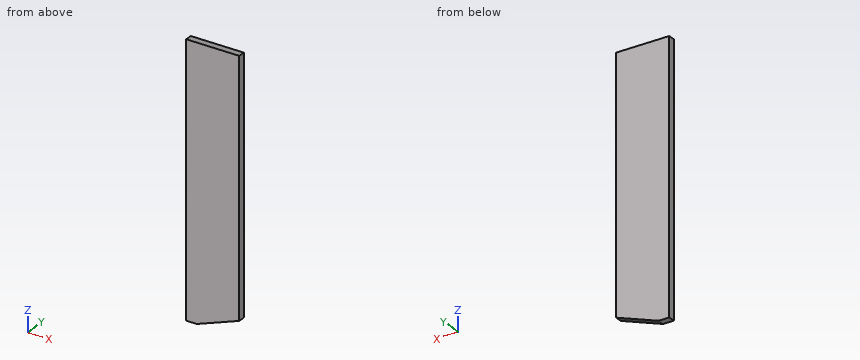
from build123d import *

# Parameters (mm, degrees)
PAD_DEPTH     = 6.5
CHAMFER_ANGLE = 20
CHAMFER_SIZE  = 80


with BuildPart() as part:
    # Sketch → Pad (new body, symmetric)
    with BuildSketch(Plane.XZ):
        Polygon((0, 0), (100, 0), (100, 500), (0, 500), (0, 1), align=None)
    extrude(amount=PAD_DEPTH, both=True)

    # Chamfer
    chamfer_edges = [part.edges().sort_by_distance(p)[0] for p in [
        (100, 0, 0),
    ]]
    chamfer_side = part.faces().sort_by_distance((50, 0, 0))[0]
    chamfer(chamfer_edges, length=CHAMFER_SIZE, angle=CHAMFER_ANGLE, reference=chamfer_side)


solid = part.part
Read the model definition and answer for the solid it produces. Units are mm, in the model's axes. Give positions to 0.01 mm unless a question says otherwise; leave off trailing zeros. Loops run counter-clockwise (first coordinate to the right, second up) from the corner with the lowest first, then second, coordinate; pieces in that order, holes last. Notation, with made-up numbers: (25, -33.5) -> (76, -33.5) arc R30 ccw to (76, 2.5) -> close; hole circle Ø10 at (80.5, 18.25). An arc over 180 degrees is marked (long way). Answer as CSV lines item,"result".
Item 1: Consider line 1 (Z direction, x = 68.5, y = -3); line 2 (Z direction, x = 28.5, y = -1). Determine where each line is inside the solid, lowest interval first. Write a range as [from, to].
Returned:
line 1,"z = [17.65, 500]"
line 2,"z = [3.09, 500]"
Item 2: Find section A-A on y = -0.25. Give the vertices of the cut face in (x, z), plus the area to 3 significant figures.
Returned:
outline,"(0, 0) -> (20, 0) -> (100, 29.12) -> (100, 500) -> (0, 500) -> close"
area,"48,800 mm²"
Item 3: Find section B-B on x = 85.5. Give the vertices of the cut face in (y, z), plus the area to 3 significant figures.
Returned:
outline,"(-6.5, 23.84) -> (6.5, 23.84) -> (6.5, 500) -> (-6.5, 500) -> close"
area,"6,190 mm²"
